from build123d import *

# Parameters (mm, degrees)
BOSS_EXTRUDE1_DEPTH          = 12.7
SERVO_HOLE_DEPTH             = 224.084518592
SERVO_HOLE_DEPTH_BACK        = 224.084518592
SKETCH3_W                    = 25.4
SKETCH3_H                    = 25.4
FILLET1_R                    = 6.35
CUT_EXTRUDE1_DEPTH           = 224.084518592
CUT_EXTRUDE1_TAPER           = -7
CUT_EXTRUDE1_OTHER_WAY_DEPTH = 224.084518592


with BuildPart() as part:
    # Sketch1 → Boss-Extrude1 (new body)
    with BuildSketch(Plane(origin=(0, 0, 0), x_dir=(1, 0, 0), z_dir=(0, 1, 0))):
        Polygon((128.31424077, 139.7), (37.592, 0), (150.368, 0), (173.46274077, 139.7), align=None)
        Polygon((113.26474077, 139.7), (0, 0), (37.592, 0), (128.31424077, 139.7), align=None)
    extrude(amount=BOSS_EXTRUDE1_DEPTH)

    # Sketch3 → servo hole (cut, two sides: drawn at the far end of the back side and taken through both)
    with BuildSketch(Plane(origin=(0, 12.7, 0), x_dir=(1, 0, 0), z_dir=(0, 1, 0)).offset(-SERVO_HOLE_DEPTH_BACK)):
        with Locations((104.447870385, 62.23)):
            Rectangle(SKETCH3_W, SKETCH3_H)
    extrude(amount=SERVO_HOLE_DEPTH + SERVO_HOLE_DEPTH_BACK, mode=Mode.SUBTRACT)

    # Fillet1
    fillet1_edges = [part.edges().sort_by_distance(p)[0] for p in [
        (56.632370385, 0, -69.85),
        (56.632370385, 12.7, -69.85),
    ]]
    fillet(fillet1_edges, radius=FILLET1_R - 0.0001)  # a hair under: the kernel refuses the full size

    # Sketch4 → Cut-Extrude1 (cut)
    with BuildSketch(Plane(origin=(0, 0, -139.7), x_dir=(-1, 0, 0), z_dir=(0, 0, -1))):
        Polygon((-134.139610484, 0), (-138.66474077, 6.35), (-134.139610484, 12.7), (-173.46274077, 12.7), (-173.46274077, 0), align=None)
    extrude(amount=-CUT_EXTRUDE1_DEPTH, taper=CUT_EXTRUDE1_TAPER, mode=Mode.SUBTRACT)

    # Sketch4 → Cut-Extrude1 other way (cut)
    with BuildSketch(Plane(origin=(0, 0, -139.7), x_dir=(-1, 0, 0), z_dir=(0, 0, -1))):
        Polygon((-134.139610484, 0), (-138.66474077, 6.35), (-134.139610484, 12.7), (-173.46274077, 12.7), (-173.46274077, 0), align=None)
    extrude(amount=CUT_EXTRUDE1_OTHER_WAY_DEPTH, mode=Mode.SUBTRACT)


solid = part.part
Work out the finished part from the listing and answer in its coordinate system (mm). A direction names the side the tool comes from. Coordinates: 2 decimals unless noted, no trailing zeros. Write item = value, one per line.
1. For faces 5 (the face through (58.9, 1.8, -69.6)), 6 (the face through (117.148, 6, -62)), determine the directions among +Z, -Z, +X, -X, +Y, -Y from which every point of the face is accessible in a straight line to the end or side of a thin tool.
Solution:
face_5 = -Z, -X, -Y
face_6 = +Y, -Y
2. Determine the mould class of faces 1 (the face through (126, 6, -139.7)), 2 (the face through (58, 6, 0)), 3 (the face through (91.748, 6, -62)), 4 (the face through (104, 6, -49.53)) for opening direction Z: released by +Z, released by -Z, zero draft, split by the parting line, or undercut.
Solution:
face_1 = released by -Z
face_2 = released by +Z
face_3 = undercut
face_4 = undercut
3. Flat-ended cylindrical pins translate along their axes: pin 1 (2 mm diameter, centred on x = 83.5, y = 5, fed in from -Z); pin 2 (3 mm diameter, centred on x = 49, y = 4.5, fed in from +Z); pin 3 (3 mm diameter, centred on y = 8.5, z = -46.5, fed in from -X). Find the tip coordinate at first contact, or state that the pin passes through.
Solution:
pin_1 = -104.03
pin_2 = 0
pin_3 = 36.83
4. Straight lines are drawn through the part: line 1 (Z direction, x = 94, y = 11); line 2 (X direction, y = 6.25, z = -63); line 3 (Z direction, x = 94, y = 8.25). For each, find the intervals that lie inside material, in ascending order. Write a range as from..to.
Solution:
line_1 = -112.72..-74.93, -49.53..0
line_2 = 51.08..91.75, 117.15..127.03
line_3 = -115.48..-74.93, -49.53..0
